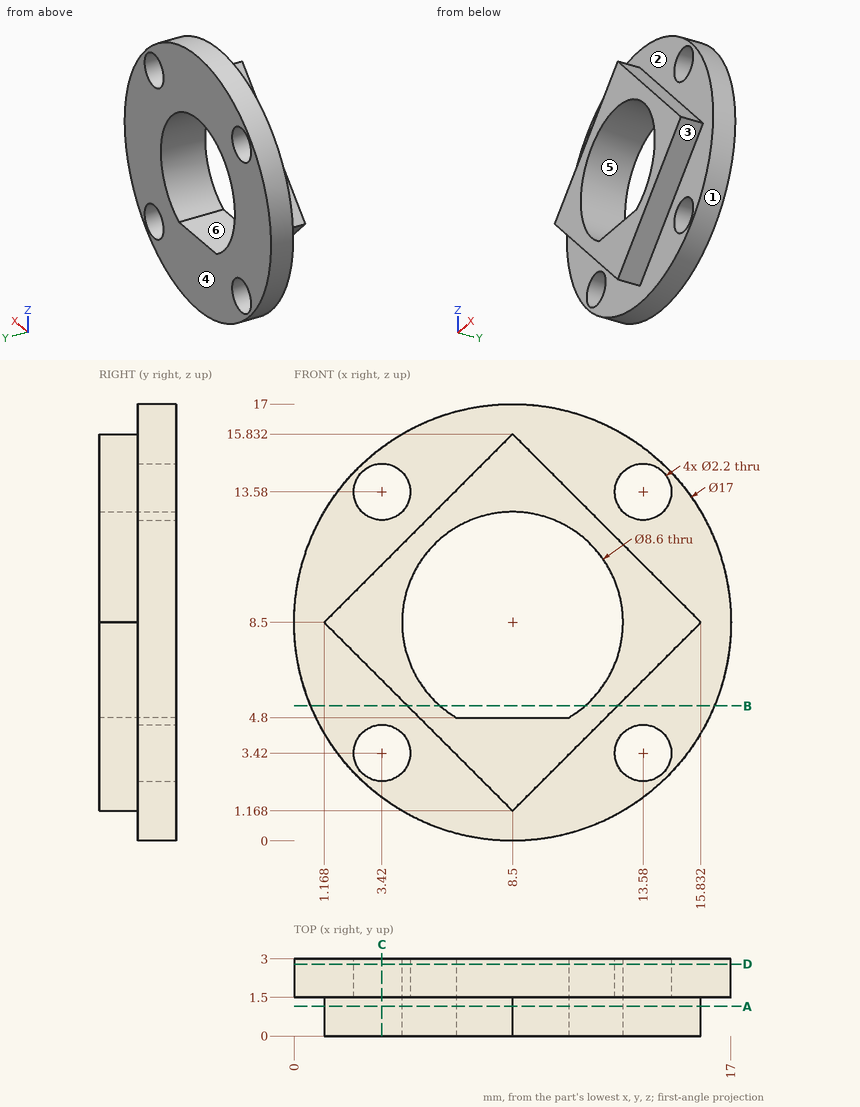
Print and shaded views of the part. All mm, measured from the part's lowest x, y and z. A direction names the side the tool comes from. Give positions to 0.01 mm unless a question says otherwise; leave off trailing zeros. Write each loop counter-clockwise with the first axis right and the second up, starting at its lowest first coordinate (ties: lowest second). Pieces come first, ordered by that corner, then holes. Notation, with made-up numbers: (-33, 59) -> (24, 59) arc R21 cw to (24, 96) -> close; hole circle Ø5 at (-16.75, -36). An arc over 180 degrees is marked (long way). Use CSV: the item, a comma, the result in double quotes. Start each with the question number.
1) Two-plate mould, pull along X, no slides. Class the marked faces 3, 4, 5 and 6: released by +X, released by -X, zero draft, split by the parting line, or undercut.
2) Drill centre lines: L1, parallel to Z at x = 13.58, y = 2.6 (1 decimal); L2, parallel to X at y = 1.1, z = 6; L3, parallel to X at y = 1.75, z = 13.25. Where is each one in solid material? Low to high.
3) Pin check, flat tips, straight feed: P1, Ø2.5, axis at x = 13.58, z = 13.58, coming from the -Y side; P2, Ø1.5, axis at x = 9.5, y = 2.5, coming from the -Z side; P3, Ø1, axis at y = 2, z = 11.5, coming from the -X side. Stop position of each tip, or through.
4) Cut at C-C on x = 3.42. List the corners of the cut face in (y, z) (1 decimal), plus the area to 3 significant figures.
5) Cut at A-A on y = 1.15. List the corners of the cut face in (x, z).
6) Cut at B-B on z = 5.25. List the corners of the cut face in (x, y) (1 decimal).
7) Tool access for the marked faces 1 and 2: list every direction of +Z, -Z, +X, -X, +Y, -Y with a clear straight run to the whole face (end or side of a thin tool).
8) Cut at D-D on y = 2.8. List the corners of the cut face in (x, z).
Final values:
1,face 3,"released by +X"
1,face 4,"zero draft"
1,face 5,"undercut"
1,face 6,"undercut"
2,L1,"z = 1.7 to 2.3, 4.5 to 12.5, 14.7 to 15.3"
2,L2,"x = 3.67 to 5, 12 to 13.33"
2,L3,"x = 1.45 to 2.37, 4.47 to 12.53, 14.63 to 15.55"
3,P1,"stops at y = 1.5"
3,P2,"stops at z = 0"
3,P3,"stops at x = 0.38"
4,outline,"(0, 6.2) -> (1.5, 6.2) -> (1.5, 4.5) -> (3, 4.5) -> (3, 12.5) -> (1.5, 12.5) -> (1.5, 10.8) -> (0, 10.8) -> close; (1.5, 1.7) -> (3, 1.7) -> (3, 2.3) -> (1.5, 2.3) -> close; (1.5, 14.7) -> (3, 14.7) -> (3, 15.3) -> (1.5, 15.3) -> close"
4,area,"20.6 mm2"
5,outline,"(1.17, 8.5) -> (8.5, 1.17) -> (15.83, 8.5) -> (8.5, 15.83) -> close; hole (6.31, 4.8) -> (10.69, 4.8) arc R4.3 ccw (long way) to start"
6,outline,"(0.6, 1.5) -> (4.4, 1.5) -> (4.4, 0) -> (5.7, 0) -> (5.7, 3) -> (0.6, 3) -> close; (11.3, 0) -> (12.6, 0) -> (12.6, 1.5) -> (16.4, 1.5) -> (16.4, 3) -> (11.3, 3) -> close"
7,face 1,"+Y, -Y"
7,face 2,"-Y"
8,outline,"circle Ø17 at (8.5, 8.5); hole circle Ø2.2 at (3.42, 3.42); hole circle Ø2.2 at (3.42, 13.58); hole (6.31, 4.8) -> (10.69, 4.8) arc R4.3 ccw (long way) to start; hole circle Ø2.2 at (13.58, 3.42); hole circle Ø2.2 at (13.58, 13.58)"
